Here's the drawing with two shaded views (mm, measured from the low corner). I have some questions. Coordinates: 2 decimals unless noted, no trailing zeros. Write each loop counter-clockwise with the first axis right and the second up, starting at its lowest first coordinate (ties: lowest second). Pieces come first, ordered by that corner, then holes.
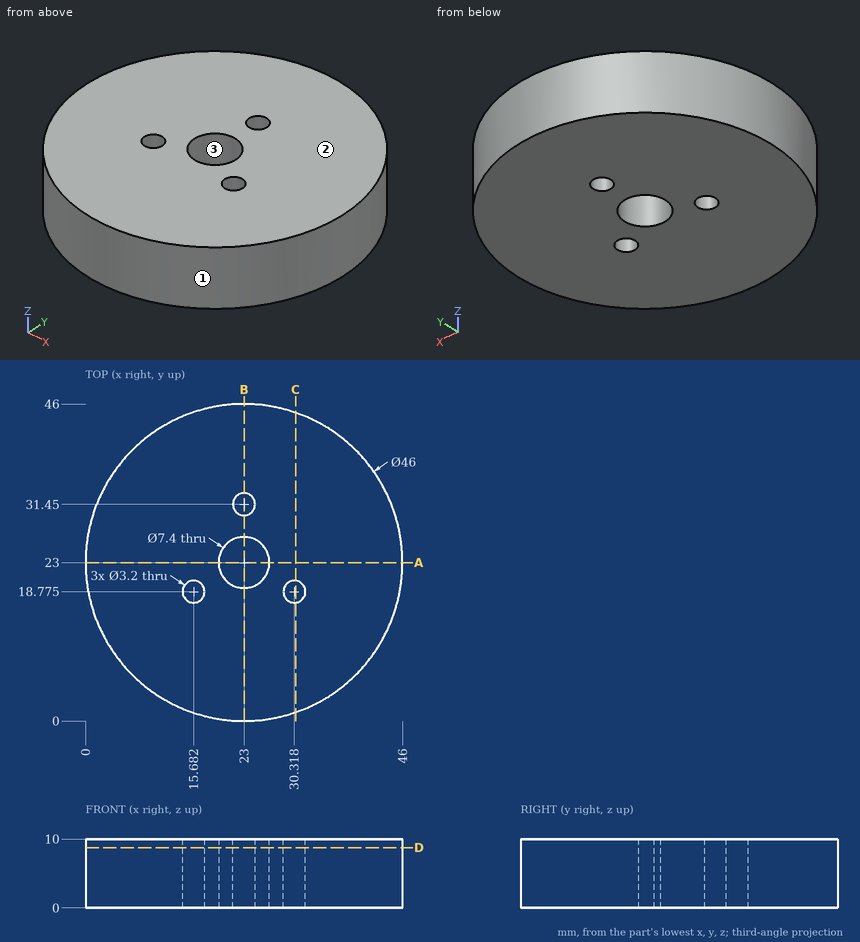
1. I want a section at D-D on z = 8.75. Please give me the cut outline in (x, y) (3 decimals), plus the area to 3 significant figures.
Verdict:
outline: circle Ø46 at (23, 23); hole circle Ø3.2 at (15.682, 18.775); hole circle Ø7.4 at (23, 23); hole circle Ø3.2 at (23, 31.45); hole circle Ø3.2 at (30.318, 18.775)
area: 1,590 mm2
2. I want a section at B-B on x = 23. Please give me the cut outline in (y, z), plus the area to 3 significant figures.
Verdict:
outline: (0, 0) - (19.3, 0) - (19.3, 10) - (0, 10) - close; (26.7, 0) - (29.85, 0) - (29.85, 10) - (26.7, 10) - close; (33.05, 0) - (46, 0) - (46, 10) - (33.05, 10) - close
area: 354 mm2
3. Please list where these lines run through material, in increasing order: line 1 along Y through (x, z) = (23, 7.75); line 2 along Y through (x, z) = (24, 6.5); line 3 along X through (y, z) = (31.5, 5).
Verdict:
line 1: y = 0 to 19.3, 26.7 to 29.85, 33.05 to 46
line 2: y = 0.02 to 19.44, 26.56 to 30.2, 32.7 to 45.98
line 3: x = 1.63 to 21.4, 24.6 to 44.37
4. If we mould it in two halves opening along Y, with no side actions, what happens to the marked faces 1, 2 and 3? For each: pulls with the +Y half, pulls with the -Y half, needs draft (parallel to the pull), parting line crosses it, or undercut.
Verdict:
face 1: parting line crosses it
face 2: needs draft
face 3: undercut
5. I want a section at C-C on x = 30.5. Please give me the cut outline in (y, z).
Verdict:
outline: (1.26, 0) - (17.19, 0) - (17.19, 10) - (1.26, 10) - close; (20.36, 0) - (44.74, 0) - (44.74, 10) - (20.36, 10) - close
6. I want a section at A-A on y = 23. Please give me the cut outline in (x, z).
Verdict:
outline: (0, 0) - (19.3, 0) - (19.3, 10) - (0, 10) - close; (26.7, 0) - (46, 0) - (46, 10) - (26.7, 10) - close
7. For pin 1 (6 mm diameter, centred on y = 31.5, z = 5, fed in from -X); pin 2 (4 mm diameter, centred on x = 32.5, y = 25.5, fed in from -Z); pin 3 (1 mm diameter, centred on x = 9.5, z = 1.5, fed in from +Y); pin 4 (1.5 mm diameter, centred on x = 15.5, z = 3, fed in from +Y), each with a flat end and sliding along its axis, tell me the tip position at first contact or that it passes through.
Verdict:
pin 1: stops at x = 0.67
pin 2: stops at z = 0
pin 3: stops at y = 41.97
pin 4: stops at y = 44.99
